```python
from build123d import *

# Parameters (mm, degrees)
PAD001_DEPTH            = 150
SKETCH001_R             = 7.5
PAD_DEPTH               = 15
SKETCH003_R             = 7.5
POCKET003_DEPTH         = 15
POCKET004_DEPTH         = 50
BODY004_PLACEMENT_ANGLE = 180


with BuildPart() as part:
    # Sketch002 (on DatumPlane) → Pad001 (new body, symmetric)
    with BuildSketch(Plane(origin=(0, -50, 50), x_dir=(0.8164965809, -0.4082482905, -0.4082482905), z_dir=(-0.5773502692, -0.5773502692, -0.5773502692))):
        Polygon((0, 0), (0, 55.7106781187), (-8.6602540378, 55.7106781187), (-40.8248290464, 0), align=None)
    extrude(amount=PAD001_DEPTH, both=True)

    # Sketch001 (on Face7 of Binder001) → Pad (join)
    with BuildSketch(Plane(origin=(0, -50, 50), x_dir=(1, 0, 0), z_dir=(0, -0.7071067812, 0.7071067812))):
        with Locations((32.1969593942, 80.8887157017)):
            Circle(SKETCH001_R)
    extrude(amount=-PAD_DEPTH)

    # Sketch003 (on Face6 of Pad) → Pocket003 (cut)
    with BuildSketch(Plane(origin=(-25, -50, 75), x_dir=(-0.4082482905, 0.8164965809, -0.4082482905), z_dir=(-0.7071067812, 0, 0.7071067812))):
        with Locations((-11.7521604853, -47.4562863756)):
            Circle(SKETCH003_R)
    extrude(amount=-POCKET003_DEPTH, mode=Mode.SUBTRACT)

    # Sketch005 (on Face6 of Pocket003) → Pocket004 (cut)
    with BuildSketch(Plane(origin=(-25, -50, 75), x_dir=(-0.4082482905, 0.8164965809, -0.4082482905), z_dir=(-0.7071067812, 0, 0.7071067812))):
        Polygon((20.4124145232, -103.8675134595), (-48.2468625128, -128.1422336512), (-48.2468625128, -150), (20.4124145232, -150), align=None)
    extrude(amount=-POCKET004_DEPTH, mode=Mode.SUBTRACT)


with BuildPart() as part_1:
    # Body004 placement: moved
    add(part.part.rotate(Axis((0, 0, 0), (0, 0, 1)), BODY004_PLACEMENT_ANGLE))


solid = part_1.part
```
Source: CAD feature listing. Evaluate the final solid. Frame: model axes, mm. A direction names the side the tool comes from. Coordinates: 2 decimals unless noted, no trailing zeros. Order: outer loops, then holes, each group sorted by start corner. A loop starts at its lowest first (then second) coordinate and runs counter-clockwise, first axis right, second up. Notation, with made-up numbers: M 32.5,6.5 L 41.5,6.5 A25 cw 41.5,29.5 Z; hole C 21,17.5 d6. An arc over 180 degrees is marked long. Write each question's results on one line, items separated by ' | '. Start each with the question number.
1) Section query A-A (x = -32.5). Return the cut outline in (y, z).
2) Contact query for flat-ended pins moving along their axis: pin 1 Ø4 at (x, y) = (-31.5, 53.5) entering from +Z; pin 2 Ø2 at (x, y) = (-28.5, 62) entering from +Z; pin 3 Ø1 at (x, y) = (6.5, 97.5) entering from +Z. Output: stop coordinate, or through.
3) Access query for faces 4 (the face through (7.43, 76.85, 61.99)), 5 (the face through (-17.786, 32.343, 96.572)). Directions: +Z, -Z, +X, -X, +Y, -Y. A direction counts if a zero-diameter tool reaches every point of the face in a straight line with its end or side. Return the directions, or none.
4) Section query C-C (z = 32.5). Return the cut outline in (x, y).
5) Line query: line 1 (Z direction, x = 105.5, y = 140); line 2 (X direction, y = 19, z = 152); line 3 (Z direction, x = 98.5, y = 102). Output: solid intervals per line, ascending. Write a range as from..to.
6) Section query B-B (y = 154). Return the cut outline in (x, z), plus the area to 3 significant figures.
7) Draft query along Z for faces 1 (the face through (-11.26, 24.88, 100.8)), 2 (the face through (10.92, 95.084, 83.703)), 3 (the face through (99.8, 145.6, -14.41)). Return one class per face: released by +Z, released by -Z, zero draft, split by the parting line, or undercut.
Answers:
1) outline: M -24.68,124.68 L -12.5,112.5 L -23.1,101.89 L -12.5,91.29 L -1.9,101.9 L 17.5,82.5 L 56.89,121.89 L 46.29,132.5 L -20.77,132.5 Z
2) pin 1: stops at z = 127.29 | pin 2: stops at z = 117.78 | pin 3: passes through
3) face 4: -Z, -X, +Y | face 5: none
4) outline: M 17.5,67.5 L 67.5,67.5 L 67.5,146.29 L 56.89,146.29 Z
5) line 1: z = -14.31..-5.5 | line 2: x = -66.5..-52 | line 3: z = -2..1.5
6) outline: M 64.61,24.79 L 86.6,-19.21 L 102.9,-2.9 L 75.21,24.79 Z | area: 685 mm^2
7) face 1: undercut | face 2: released by +Z | face 3: released by -Z
